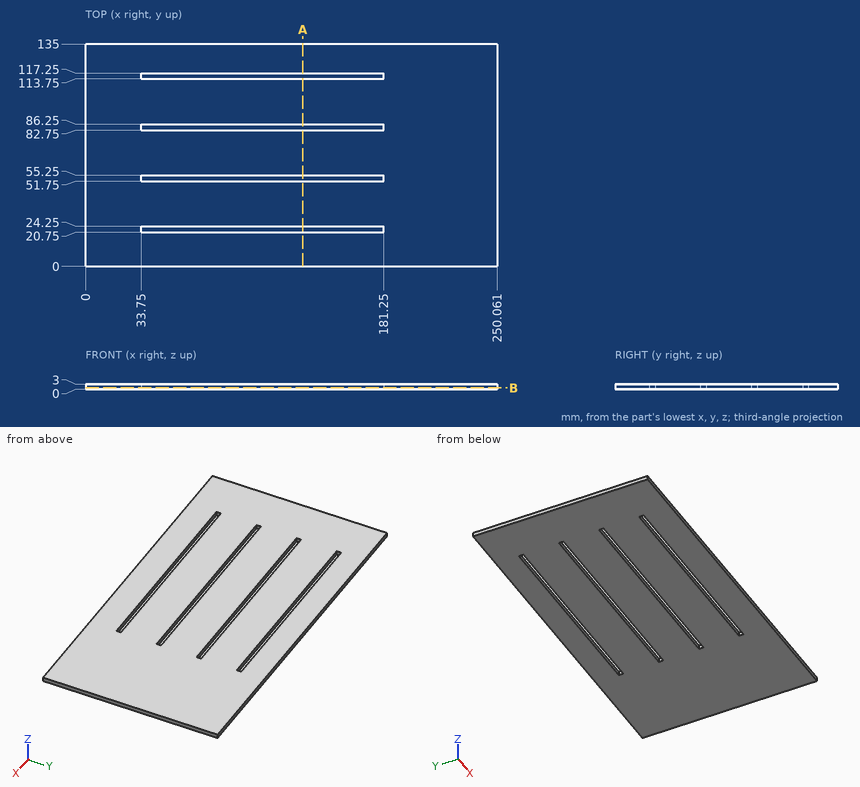
Check sheet for the drawn part. Datum: minimum x, y, z corner. Units: mm. Round coordinates to 2 decimals unless told otherwise and drop trailing zeros. Order: outer loops, then holes, each group sorted by start corner. A loop starts at its lowest first (then second) coordinate and runs counter-clockwise, first axis right, second up.
1) Section check A-A (x = 132). Record the boundary of the cut face in (y, z), and give its area (3 significant figures).
2) Scan lines: line 1 (Y direction, x = 72, z = 0.4); line 2 (X direction, y = 115.5, z = 1.4). Record each from-to range of solid material in increasing order.
3) Section check B-B (z = 0.85). Record the boundary of the cut face in (x, y).
Result:
1. outline: (0, 0) - (20.75, 0) - (20.75, 3) - (0, 3) - close; (24.25, 0) - (51.75, 0) - (51.75, 3) - (24.25, 3) - close; (55.25, 0) - (82.75, 0) - (82.75, 3) - (55.25, 3) - close; (86.25, 0) - (113.75, 0) - (113.75, 3) - (86.25, 3) - close; (117.25, 0) - (135, 0) - (135, 3) - (117.25, 3) - close
1. area: 363 mm2
2. line 1: y = 0 to 20.75, 24.25 to 51.75, 55.25 to 82.75, 86.25 to 113.75, 117.25 to 135
2. line 2: x = 0 to 33.75, 181.25 to 250.06
3. outline: (0, 0) - (250.06, 0) - (250.06, 135) - (0, 135) - close; hole (33.75, 20.75) - (181.25, 20.75) - (181.25, 24.25) - (33.75, 24.25) - close; hole (33.75, 51.75) - (181.25, 51.75) - (181.25, 55.25) - (33.75, 55.25) - close; hole (33.75, 82.75) - (181.25, 82.75) - (181.25, 86.25) - (33.75, 86.25) - close; hole (33.75, 113.75) - (181.25, 113.75) - (181.25, 117.25) - (33.75, 117.25) - close
